Read the model definition and answer for the solid it produces. Units are mm, in the model's axes. A direction names the side the tool comes from. Give positions to 0.01 mm unless a question says otherwise; leave off trailing zeros. Loops run counter-clockwise (first coordinate to the right, second up) from the corner with the lowest first, then second, coordinate; pieces in that order, holes last.
(1) Find section D-D, the plane y = 42.5. Write down the section's boundary in (x, z).
(2) Each of these flat-tipped pins is pushed along its axis until it touches: P1, Ø1.1, axis at x = -39.5, z = -2.5, coming from the -Y side; P2, Ø1.1, axis at x = -26, z = -1, coming from the -Y side; P3, Ø7, axis at x = 14.5, y = 11.5, coming from the +Z side; P4, Ø5.5, axis at x = -13.67, y = 10.11, coming from the +Z side. Where does it stop, or does it pass through?
(3) Determine the mould class of faces 1 (the face through (0, -10.644, -2)), 2 (the face through (42.326, 23, -2)), 3 (the face through (-11.9, 2.4, -1.8)) for opening direction X: pulls with the +X half, pulls with the -X half, needs draft (parallel to the pull), parting line crosses it, or undercut.
(4) Find section B-B, the plane z = -1.1. State how many separate pieces and enclosed holes the cut face has, then the cut area to 3 significant figures.
(5) Find section A-A, the plane y = 6. Write down the section's boundary in (x, z).
(6) Straight lines are drawn through the part: probe 1 along Y at (x, z) = (1.5, -2.8); probe 2 along Y at (x, z) = (-4.5, -0.55); probe 3 along X at (y, z) = (18.5, -2.6). For each, find the intervals that lie inside material, in ascending order.
(7) Which of the six approach directions +Z, -Z, +X, -X, +Y, -Y give full straight-line access (tool end or side, diameter ignored) to faces 4 (the face through (-16.845, 10.245, -1.726)), 5 (the face through (22.852, -5, -2)), 6 (the face through (-22.198, -5, -2)), 7 (the face through (-39, 35.286, -2)), 8 (the face through (36.242, 40, -2))?
(8) Find section C-C, the plane x = -34. Write down the section's boundary in (y, z), then the cut area to 4 significant figures.
Autodesk Inventor part; units mm, degrees
ref_plane "YZ Plane" through (0, 0, 0) normal (1, 0, 0) x (0, 1, 0)
ref_plane "XZ Plane" through (0, 0, 0) normal (0, 1, 0) x (-1, 0, 0)
ref_plane "XY Plane" through (0, 0, 0) normal (0, 0, 1) x (1, 0, 0)
sketch "Sketch1" plane through (0, 0, 0) normal (0, 0, 1) x (1, 0, 0)
  line L0 (-22.1985, -10.6442) -> (22.8515, -10.6442)
  line L1 (22.8515, -10.6442) -> (22.8515, 0.6058)
  line L2 (22.8515, 0.6058) -> (32.8515, 0.6058)
  line L3 (32.8515, 0.6058) -> (32.8515, 45.6058)
  line L4 (32.8515, 45.6058) -> (-32.1985, 45.6058)
  line L5 (-32.1985, 45.6058) -> (-32.1985, 0.6058)
  line L6 (-32.1985, 0.6058) -> (-22.1985, 0.6058)
  line L7 (-22.1985, 0.6058) -> (-22.1985, -10.6442)
  point P0 (0, 0)
  dimension "d0" = 45.05
  dimension "d1" = 11.25
  dimension "d2" = 10
  dimension "d3" = 45
  dimension "d4" = 45
  dimension "d5" = 10
  dimension "d6" = 65.05
extrude "Extrusion1" add sketch "Sketch1" against normal blind 3.7
sketch "Sketch2" plane through (0, 0, 0) normal (0, 0, 1) x (1, 0, 0)
  point P0 (0, 0)
sketch "Sketch3" plane through (0, 0, 0) normal (0, 0, 1) x (1, 0, 0)
  circle A0 centre (0.3265, 10.1058) radius 6.05
  line L0 (-32.1985, 45.6058) -> (-32.1985, 0.6058)
  line L1 (-32.1985, 0.6058) -> (-22.1985, 0.6058)
  circle A1 centre (14.3265, 10.1058) radius 3.175
  circle A2 centre (-13.6735, 10.1058) radius 3.175
  circle A3 centre (0.3265, 10.1058) radius 15.5
  circle A4 centre (0.3265, 25.6058) radius 1.75
  circle A5 centre (0.3265, -5.3942) radius 1.5
  line L2 (32.8515, 0.6058) -> (32.8515, 45.6058)
  circle A6 centre (-12.9494, 18.1058) radius 1.75
  circle A7 centre (-13.5028, 3.1058) radius 1.75
  circle A8 centre (14.1558, 3.1058) radius 1.75
  circle A9 centre (13.6024, 18.1058) radius 1.75
  circle A10 centre (0.3265, 10.1058) radius 18.5
  point P0 (0, 0)
  dimension "d9" = 12.1
  dimension "d10" = 32.525
  dimension "d11" = 9.5
  dimension "d12" = 6.35
  dimension "d13" = 14
  dimension "d14" = 6.35
  dimension "d15" = 14
  dimension "d20" = 31
  dimension "d21" = 3.5
  dimension "d22" = 32.525
  dimension "d23" = 3
  dimension "d24" = 32.525
  dimension "d25" = 3.5
  dimension "d26" = 8
  dimension "d27" = 3.5
  dimension "d28" = 3.5
  dimension "d29" = 3.5
  dimension "d30" = 8
  dimension "d31" = 15
  dimension "d36" = 37
  dimension "d54" = 15
extrude "Extrusion2" cut sketch "Sketch3" against normal blind 5 contours A0
sketch "Sketch4" plane through (0, 0, 0) normal (0, 0, 1) x (1, 0, 0)
  point P0 (0, 0)
extrude "Extrusion4" cut sketch "Sketch3" against normal blind 3.5 contours A1 A3 | A3 A1 | A3 A2 | A2 A3
extrude "Extrusion5" cut sketch "Sketch3" against normal blind 5 contours A9 A3 | A3 A9 | A8 A3 | A3 A8 | A4 A3 | A3 A4 | A5 A3 | A3 A5 | A6 A3 | A3 A6 | A7 A3 | A3 A7
sketch "Sketch5" plane through (0, 0, 0) normal (0, 0, 1) x (1, 0, 0)
  point P0 (0, 0)
sketch "Sketch6" plane through (0, 0, 0) normal (0, 0, 1) x (1, 0, 0)
  line L0 (-35.5885, 45.6058) -> (-32.1985, 45.6058)
  line L1 (-32.1985, 45.6058) -> (-32.1985, 0.6058)
  line L2 (-32.1985, 0.6058) -> (-35.5885, 0.6058)
  line L3 (-35.5885, 0.6058) -> (-35.5885, 45.6058)
  line L4 (-32.1985, 45.6058) -> (-32.1985, 0.6058)
  line L5 (32.8515, 45.6058) -> (-32.1985, 45.6058)
  line L6 (-32.1985, 0.6058) -> (-22.1985, 0.6058)
  line L7 (32.8515, 45.6058) -> (32.8515, 0.6058)
  line L8 (32.8515, 0.6058) -> (32.8515, 45.6058)
  line L9 (32.8515, 0.6058) -> (36.2415, 0.6058)
  line L10 (36.2415, 0.6058) -> (36.2415, 45.6058)
  line L11 (36.2415, 45.6058) -> (32.8515, 45.6058)
  line L12 (22.8515, 0.6058) -> (32.8515, 0.6058)
  point P0 (0, 0)
  dimension "d37" = 0
  dimension "d38" = 0
  dimension "d39" = 0
  dimension "d40" = 3.39
  dimension "d41" = 3.39
  dimension "d42" = 0
  dimension "d43" = 0
  dimension "d44" = 0
extrude "Extrusion6" add sketch "Sketch6" against normal blind 3.7
sketch "Sketch7" plane through (0, 0, 0) normal (0, 0, 1) x (1, 0, 0)
  line L0 (30.309, 35.2858) -> (30.309, 10.9258)
  line L1 (30.309, 10.9258) -> (42.3265, 10.9258)
  line L2 (42.3265, 10.9258) -> (42.3265, 35.2858)
  line L3 (42.3265, 35.2858) -> (30.309, 35.2858)
  line L4 (36.2415, 45.6058) -> (-35.5885, 45.6058)
  line L5 (22.8515, 0.6058) -> (36.2415, 0.6058)
  line L6 (36.2415, 0.6058) -> (36.2415, 45.6058)
  line L7 (-41.6735, 35.2858) -> (-29.8249, 35.2858)
  line L8 (-29.8249, 35.2858) -> (-29.8249, 10.9258)
  line L9 (-29.8249, 10.9258) -> (-41.6735, 10.9258)
  line L10 (-41.6735, 10.9258) -> (-41.6735, 35.2858)
  line L11 (-35.5885, 0.6058) -> (-22.1985, 0.6058)
  line L12 (-35.5885, 45.6058) -> (-35.5885, 0.6058)
  point P0 (0, 0)
  point P1 (36.2415, 35.2858)
  point P2 (36.2415, 10.9258)
  point P3 (-35.5885, 10.9258)
  point P4 (-35.5885, 35.2858)
  dimension "d47" = 10.32
  dimension "d48" = 10.32
  dimension "d49" = 6.085
  dimension "d50" = 10.32
  dimension "d51" = 6.085
extrude "Extrusion7" add sketch "Sketch7" against normal blind 3.7 contours L12 L9 L10 L7 | L3 L2 L1 L6
properties part number "pump part"
Entries:
1. outline: (-35.59, -3.7) - (36.24, -3.7) - (36.24, 0) - (-35.59, 0) - close
2. P1: stops at y = 10.93
2. P2: stops at y = 0.61
2. P3: stops at z = 0
2. P4: stops at z = -3.5
3. face 1: needs draft
3. face 2: pulls with the +X half
3. face 3: undercut
4. separate pieces: 1
4. enclosed holes: 9
4. area: 3,800 mm2
5. outline: (-35.59, -3.7) - (-4.12, -3.7) - (-4.12, 0) - (-35.59, 0) - close; (4.77, -3.7) - (36.24, -3.7) - (36.24, 0) - (4.77, 0) - close
6. probe 1: y = -10.64 to -6.33, -4.46 to 4.17, 16.04 to 24.31, 26.9 to 45.61
6. probe 2: y = -10.64 to 6.46, 13.75 to 45.61
6. probe 3: x = -41.67 to -14.65, -11.24 to 11.9, 15.31 to 42.33
7. face 4: +Z
7. face 5: +Z, -Z, +X, -Y
7. face 6: +Z, -Z, -X, -Y
7. face 7: +Z, -Z, -X, +Y
7. face 8: +Z, -Z, +X, +Y
8. outline: (0.61, -3.7) - (45.61, -3.7) - (45.61, 0) - (0.61, 0) - close
8. area: 166.5 mm2
